```python
from build123d import *

# Parameters (mm, degrees)
SKETCH1_W           = 188.7
SKETCH1_H           = 164
BOSS_EXTRUDE1_DEPTH = 12.5
SKETCH3_R           = 5
REVOLVE1_ANGLE      = 180


with BuildPart() as part:
    # Sketch1 → Boss-Extrude1 (new body)
    with BuildSketch(Plane.XY):
        with Locations((94.35, 82)):
            Rectangle(SKETCH1_W, SKETCH1_H)
    extrude(amount=BOSS_EXTRUDE1_DEPTH)

    # Sketch3 → Revolve1 (revolve)
    with BuildSketch(Plane.XY.offset(12.5)):
        with Locations((66.676185661, 82)):
            Circle(SKETCH3_R)
    revolve(axis=Axis((94.35, 164, 12.5), (0, 1, 0)), revolution_arc=REVOLVE1_ANGLE)


solid = part.part
```
The model under review builds one solid part; all positions refer to its coordinate system, in mm. Give positions to 0.01 mm unless a question says otherwise; leave off trailing zeros. Write each loop counter-clockwise with the first axis right and the second up, starting at its lowest first coordinate (ties: lowest second). Pieces come first, ordered by that corner, then holes. Notation, with made-up numbers: M 28.25,-32.5 L 52.25,-32.5 A13 ccw 52.25,-12.5 Z; hole C 84.5,0 d9. An arc over 180 degrees is marked long. Write item = value, one per line. Start each with the question number.
Q1. For line 1 (Z direction, x = 138.5, y = 64); line 2 (Y direction, x = 68.5, z = 28), list the stretches that pass through material, from the lowest coordinate up.
Q2. We need section A-A (y = 16.5). State the section outline as (x, z) points, plus the area to 3 significant figures.
Q3. Clearance check with flat-ended pins moving along their axes: pin 1 (1.5 mm diameter, centred on y = 86.5, z = 19, fed in from -X); pin 2 (12 mm diameter, centred on x = 118, y = 33, fed in from +Z). State where each tip first meets the part, or that it passes through.
Q4. We need section B-B (x = 152). State the section outline as (y, z) points, plus the area to 3 significant figures.
Result set:
q1.line_1 = 0 to 12.5
q1.line_2 = 77.65 to 86.35
q2.outline = M 0,0 L 188.7,0 L 188.7,12.5 L 0,12.5 Z
q2.area = 2,360 mm2
q3.pin_1 = 64.04
q3.pin_2 = 12.5
q4.outline = M 0,0 L 164,0 L 164,12.5 L 0,12.5 Z
q4.area = 2,050 mm2
